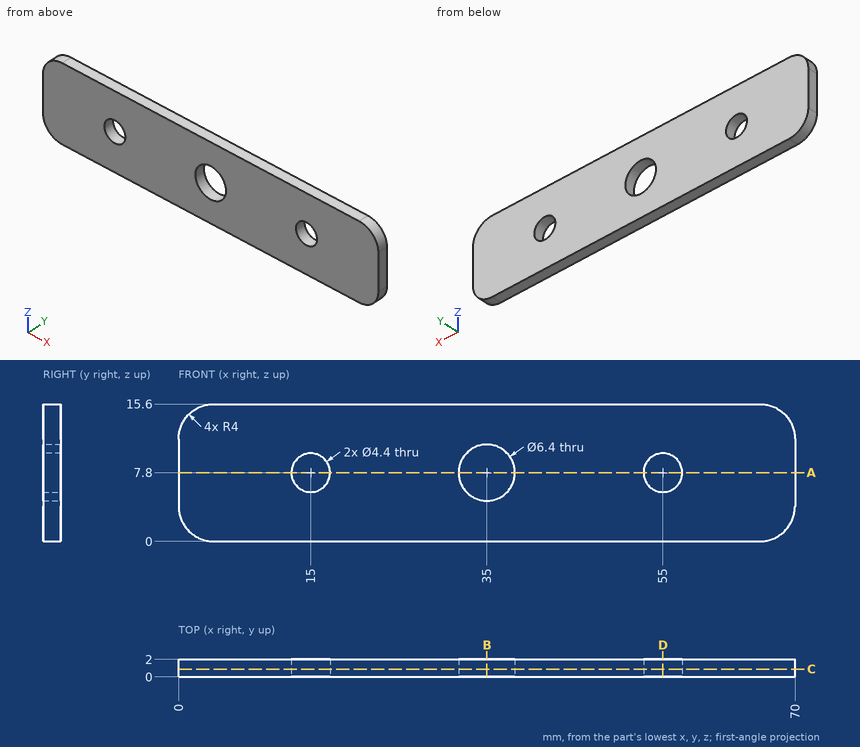
The drawing under review shows one solid part. Ordinate dimensions are in mm from its lowest x, y, z. Round coordinates to 2 decimals unless told otherwise and drop trailing zeros. Write each loop counter-clockwise with the first axis right and the second up, starting at its lowest first coordinate (ties: lowest second). Pieces come first, ordered by that corner, then holes. Notation, with made-up numbers: M 66.25,-38.5 L 78.25,-38.5 A31 cw 78.25,-6.5 Z; hole C -38.75,78.5 d10. An arc over 180 degrees is marked long. One line per item, written item: value. Start each with the question number.
(1) We need section B-B (x = 35). Give the boundary of the cut face in (y, z).
(2) We need section A-A (z = 7.8). Give the boundary of the cut face in (x, y), and give its area (3 significant figures).
(3) We need section D-D (x = 55). Give the boundary of the cut face in (y, z).
(4) Wall thickness on line 1 (X direction, y = 0.75, z = 7.8); line 2 (X direction, y = 1.95, z = 6.75); line 3 (Z direction, x = 53.5, y = 1.85): over which ranges is each line inside the solid? List them lowest first.
(5) We need section C-C (y = 0.9). Give the boundary of the cut face in (x, z).
Result:
1. outline: M 0,0 L 2,0 L 2,4.6 L 0,4.6 Z; M 0,11 L 2,11 L 2,15.6 L 0,15.6 Z
2. outline: M 0,0 L 12.8,0 L 12.8,2 L 0,2 Z; M 17.2,0 L 31.8,0 L 31.8,2 L 17.2,2 Z; M 38.2,0 L 52.8,0 L 52.8,2 L 38.2,2 Z; M 57.2,0 L 70,0 L 70,2 L 57.2,2 Z
2. area: 110 mm²
3. outline: M 0,0 L 2,0 L 2,5.6 L 0,5.6 Z; M 0,10 L 2,10 L 2,15.6 L 0,15.6 Z
4. line 1: 0 to 12.8, 17.2 to 31.8, 38.2 to 52.8, 57.2 to 70
4. line 2: 0 to 13.07, 16.93 to 31.98, 38.02 to 53.07, 56.93 to 70
4. line 3: 0 to 6.19, 9.41 to 15.6
5. outline: M 0,4 A4 ccw 4,0 L 66,0 A4 ccw 70,4 L 70,11.6 A4 ccw 66,15.6 L 4,15.6 A4 ccw 0,11.6 Z; hole C 15,7.8 d4.4; hole C 35,7.8 d6.4; hole C 55,7.8 d4.4
